Drawing for the job (mm, zero at the part's lowest x, y, z). Coordinates: 2 decimals unless noted, no trailing zeros. Loops run counter-clockwise (first coordinate to the right, second up) from the corner with the lowest first, then second, coordinate; pieces in that order, holes last.
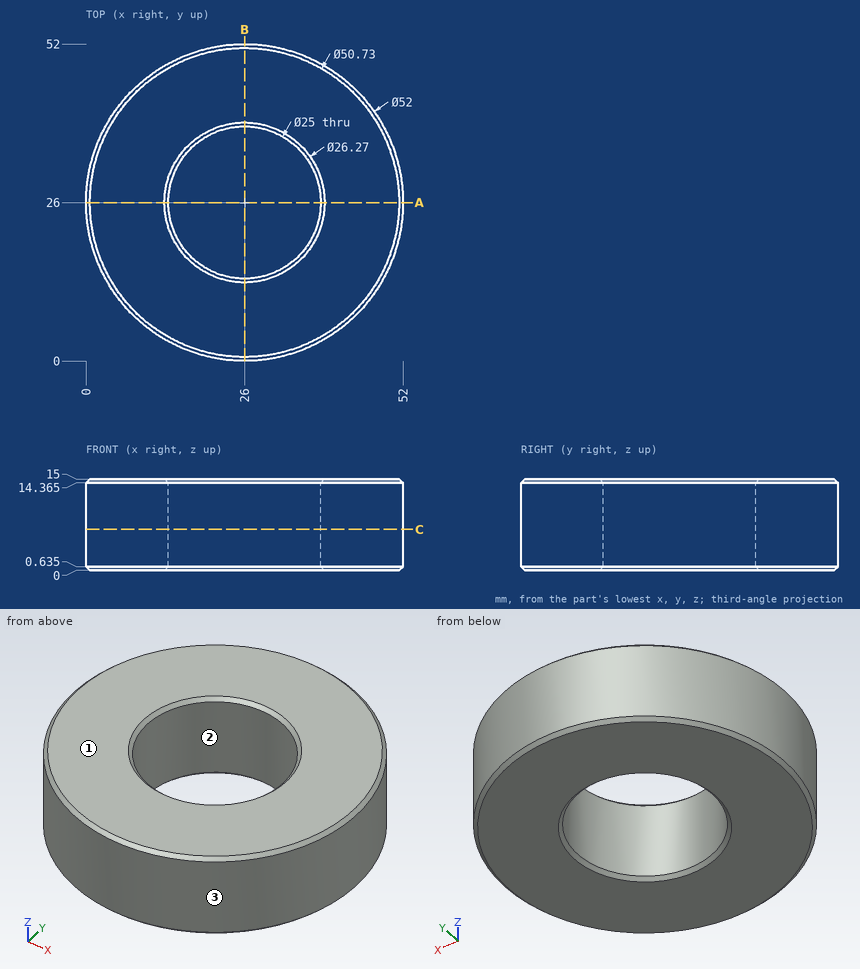
Q1. Saw through at A-A (y = 26). List the corners of the cut face in (x, z) (3 decimals).
Q2. Probe line 1 (Y direction, x = 26, z = 4.5); line 2 (X direction, y = 26.5, z = 3); line 3 (Y direction, x = 29.5, z = 6.75). List the from-to ranges inside material, lowest first.
Q3. Saw through at C-C (z = 6.75). List the corners of the cut face in (x, y).
Q4. Mould opens along X. For the marked faces 1, 2 and 3 say: released by +X, released by -X, zero draft, split by the parting line, or undercut.
Q5. Drop flat-ended pins along their axis: P1, Ø4, axis at x = 21.5, z = 11, coming from the +Y side; P2, Ø4, axis at x = 19.5, z = 7.5, coming from the +Y side; P3, Ø6, axis at y = 27, z = 3, coming from the +X side; P4, Ø4, axis at y = 38.5, z = 2, coming from the +X side. Give the stop position or say it passes through.
Checked values:
1. outline: (0, 0.635) - (0.635, 0) - (12.865, 0) - (13.5, 0.635) - (13.5, 14.365) - (12.865, 15) - (0.635, 15) - (0, 14.365) - close; (38.5, 0.635) - (39.135, 0) - (51.365, 0) - (52, 0.635) - (52, 14.365) - (51.365, 15) - (39.135, 15) - (38.5, 14.365) - close
2. line 1: y = 0 to 13.5, 38.5 to 52
2. line 2: x = 0 to 13.51, 38.49 to 52
2. line 3: y = 0.24 to 14, 38 to 51.76
3. outline: circle Ø52 at (26, 26); hole circle Ø25 at (26, 26)
4. face 1: zero draft
4. face 2: undercut
4. face 3: split by the parting line
5. P1: stops at y = 51.88
5. P2: stops at y = 51.61
5. P3: stops at x = 52
5. P4: stops at x = 49.79
